Here's how the part is built. I have some questions about the finished solid (model axes, mm). A direction names the side the tool comes from. Give positions to 0.01 mm unless a question says otherwise; leave off trailing zeros. Order: outer loops, then holes, each group sorted by start corner. A loop starts at its lowest first (then second) coordinate and runs counter-clockwise, first axis right, second up. Notation, with made-up numbers: M -23,70 L -16,70 A19 cw -16,81 Z; hole C -11.5,6.25 d1. An arc over 180 degrees is marked long. Use one line per item in the form item = value.
from build123d import *

# Parameters (mm, degrees)
EXTRUDE1_DEPTH    = 8
EXTRUDE5_DEPTH    = 8
SKETCH4_W         = 10.001997138
SKETCH4_H         = 8
EXTRUDE6_DEPTH    = 1
SKETCH2_R         = 1.5
EXTRUDE2_DEPTH    = 3
EXTRUDE7_DEPTH    = 9
SKETCH6_W         = 4.34249483
SKETCH6_H         = 6
EXTRUDE8_DEPTH    = 3
EXTRUDE9_DEPTH    = 8
CIRPATTERN1_COUNT = 7
CIRPATTERN1_ANGLE = 23.8


with BuildPart() as part:
    # Sketch1 → Extrude1 (new body)
    with BuildSketch(Plane.XY):
        with BuildLine():
            Line((0, 0), (-10, 0))
            ThreePointArc((-10, 0), (-11.85132197, -12.02823198), (-17.233918228, -22.943057454))
            Line((-17.233918228, -22.943057454), (-9.042397786, -28.678821818))
            ThreePointArc((-9.042397786, -28.678821818), (-2.314152463, -15.035289975), (0, 0))
        make_face()
    extrude(amount=EXTRUDE1_DEPTH)

    # Sketch3 → Extrude5 (add)
    with BuildSketch(Plane.XY):
        Polygon((-10, 0), (-10, 0.199866806), (0, 0), align=None)
    extrude(amount=EXTRUDE5_DEPTH)

    # Sketch4 → Extrude6 (add)
    with BuildSketch(Plane(origin=(0, 0, 0), x_dir=(-0.999800326, 0.01998269, 0), z_dir=(0.01998269, 0.999800326, 0))):
        with Locations((5.000998569, 4)):
            Rectangle(SKETCH4_W, SKETCH4_H)
    extrude(amount=EXTRUDE6_DEPTH)

    # Sketch2 → Extrude2 (cut)
    with BuildSketch(Plane(origin=(0.01998269, 0.999800326, 0), x_dir=(0.999800326, -0.01998269, 0), z_dir=(-0.01998269, -0.999800326, 0))):
        with Locations((-5.000998569, 4)):
            Circle(SKETCH2_R)
    extrude(amount=EXTRUDE2_DEPTH, mode=Mode.SUBTRACT)

    # Sketch5 → Extrude7 (cut, through all)
    with BuildSketch(Plane.XY.offset(8)):
        with BuildLine():
            Line((-0.04, -1.99959996), (-7.39025898, -1.852692681))
            ThreePointArc((-7.39025898, -1.852692681), (-9.612195577, -13.705756232), (-15.063165311, -24.46303501))
            Line((-15.063165311, -24.46303501), (-9.042397786, -28.678821818))
            Line((-9.042397786, -28.678821818), (-2.903131431, -26.123748854))
            Line((-2.903131431, -26.123748854), (1.597548849, -2.850180748))
            Line((1.597548849, -2.850180748), (-0.04, -1.99959996))
        make_face()
    extrude(amount=-EXTRUDE7_DEPTH, mode=Mode.SUBTRACT)

    # Sketch6 → Extrude8 (cut)
    with BuildSketch(Plane(origin=(-0.03996538, -1.999600652, 0), x_dir=(0.999800326, -0.01998269, 0), z_dir=(-0.01998269, -0.999800326, 0))):
        with Locations((-9.52300897, 4)):
            Rectangle(SKETCH6_W, SKETCH6_H)
    extrude(amount=EXTRUDE8_DEPTH, mode=Mode.SUBTRACT)

    # Sketch7 → Extrude9 (add)
    with BuildSketch(Plane.XY.offset(8)):
        Polygon((-15.063165311, -24.46303501), (-13.5637082, -24.827254247), (-13.037257571, -24.036463671), (-13.951792747, -22.793623096), align=None)
    extrude9 = extrude(amount=-EXTRUDE9_DEPTH)

    # CirPattern1: Extrude9 ×7 about axis
    cirpattern1_axis = Axis((-50, 0, 0), (0, 0, 1))
    for i in range(1, CIRPATTERN1_COUNT):
        add(extrude9.rotate(cirpattern1_axis, i * CIRPATTERN1_ANGLE / (CIRPATTERN1_COUNT - 1)))


solid = part.part
Q1. I want a section at B-B on z = 4.75. State how many separate pieces and enclosed holes the cut face has, then the cut area to 3 significant figures.
Found:
separate_pieces = 3
enclosed_holes = 0
area = 91.2 mm²
Q2. Thinking about a two-plate mould opening in X: for faces 1 (the face through (-12.236, -19.821, 4.056)), 2 (the face through (-11.8, -11.86, 3.94)), 3 (the face through (-9, -10, 0)), which applies, +X half, -X half, draft (parallel to the pull), parting line (faces both ways), or undercut?
Found:
face_1 = undercut
face_2 = -X half
face_3 = draft
Q3. I need wall thicknesses on L1, parallel to X at y = -17.25, z = 5; L2, parallel to Y at x = -7, z = 2.25; L3, parallel to Y at x = -13.75, z = 3.75. Which ranges of each line are inside material? Lowest first, please.
Found:
L1 = -13.91 to -10.99
L2 = -8.08 to -6.78, -1.86 to 1.14
L3 = -24.78 to -23.07, -22.47 to -16.91
Q4. I want a section at A-A on y = -3.5. Write out the boundary of the cut face in (x, z).
Found:
outline = M -10.15,0 L -7.49,0 L -7.49,1 L -10.15,1 Z; M -10.15,7 L -7.49,7 L -7.49,8 L -10.15,8 Z
Q5. I'm going to push flat-ended pins straight in: pin 1 Ø3 at (x, z) = (-4.5, 3) entering from +Y; pin 2 Ø1 at (y, z) = (-19.5, 2) entering from +X. Where does each tip first touch, or does it pass through?
Found:
pin_1 = 1.12
pin_2 = -10.22
Q6. I want a section at D-D on y = -15.5. Write out the boundary of the cut face in (x, z), then the cut area to 3 significant figures.
Found:
outline = M -13.13,0 L -9.32,0 L -9.32,8 L -13.13,8 Z
area = 30.4 mm²
Q7. On a 3-axis mill with a long thin cutter (end or side, diameter ignored), from which of +Z, -Z, +X, -X, +Y, -Y can I reach the whole of each face in a straight line? I mean faces 4 (the face through (-10.605, -18.16, 4.056)), 5 (the face through (-0.01, -1.01, 3.94)), 6 (the face through (-12.705, -22.116, 4.056)). Say none if no direction works.
Found:
face_4 = +Z, -Z, +X
face_5 = +Z, -Z, +X, -Y
face_6 = +Z, -Z
Q8. I want a section at C-C on x = -1. Write out the boundary of the cut face in (y, z), then the cut area to 3 significant figures.
Found:
outline = M -1.98,0 L 1.02,0 L 1.02,8 L -1.98,8 Z
area = 24.0 mm²
